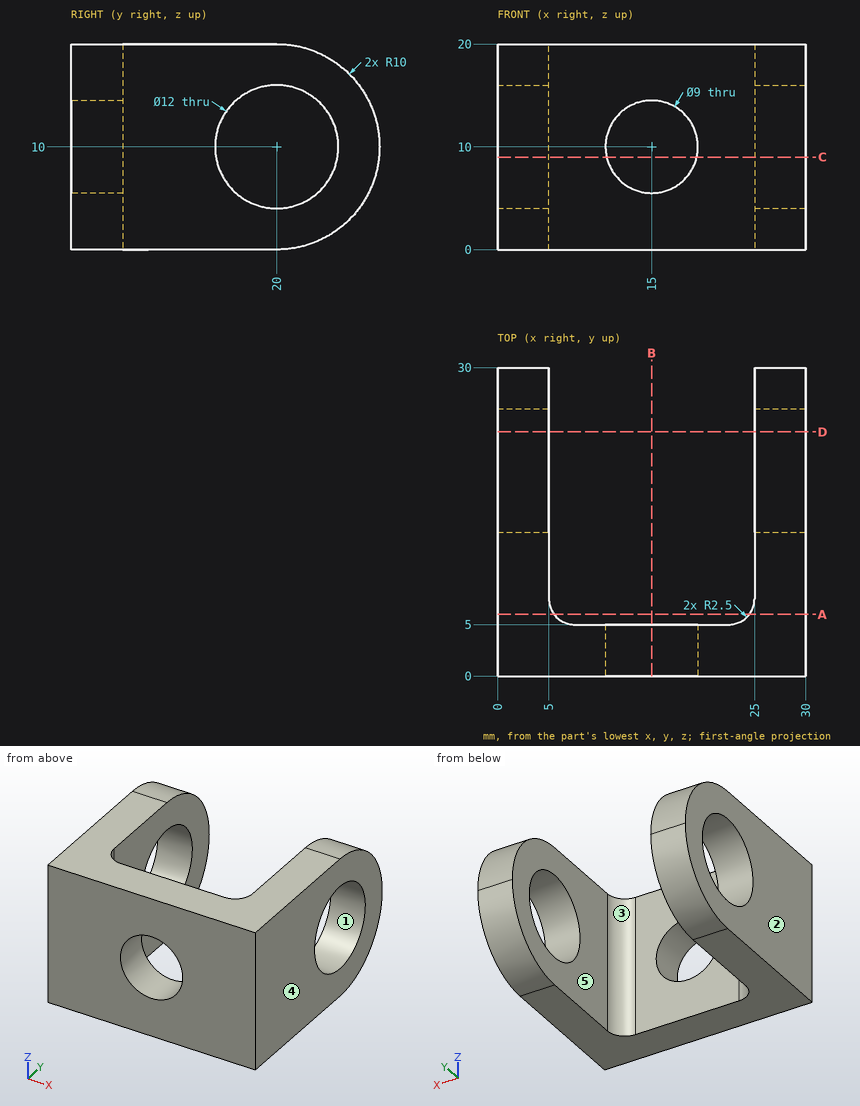
Job drawing, mm, ordinate dimensions from the low corner. One solid piece. A direction names the side the tool comes from. Give positions to 0.01 mm unless a question says otherwise; leave off trailing zeros. Write each loop counter-clockwise with the first axis right and the second up, starting at its lowest first coordinate (ties: lowest second). Pieces come first, ordered by that corner, then holes. Notation, with made-up numbers: (31, 30.25) -> (68, 30.25) arc R35 ccw to (68, 67.25) -> close; hole circle Ø7 at (-30.5, -14.75). An arc over 180 degrees is marked (long way). Return JSON: item names as keys, results as strings.
Item 1: Two-plate mould, pull along X, no slides. Class the marked faces 1, 2 and 3: +X half, -X half, draft (parallel to the pull), parting line (faces both ways), or undercut.
Answer below:
{"face 1": "draft", "face 2": "-X half", "face 3": "undercut"}
Item 2: Tool access for the marked faces 4 and 5: list every direction of +Z, -Z, +X, -X, +Y, -Y with a clear straight run to the whole face (end or side of a thin tool).
Answer below:
{"face 4": "+Z, -Z, +X, +Y, -Y", "face 5": "+Z, -Z, +Y"}
Item 3: Band-saw the part on A-A (y = 6). List the corners of the cut face in (x, z), then the cut area to 3 significant figures.
Answer below:
{"outline": "(0, 0) -> (5.5, 0) -> (5.5, 20) -> (0, 20) -> close; (24.5, 0) -> (30, 0) -> (30, 20) -> (24.5, 20) -> close", "area": "220 mm2"}
Item 4: Band-saw the part on C-C (z = 9). List the corners of the cut face in (x, y), then the cut area to 3 significant figures.
Answer below:
{"outline": "(0, 0) -> (10.61, 0) -> (10.61, 5) -> (7.5, 5) arc R2.5 cw to (5, 7.5) -> (5, 14.08) -> (0, 14.08) -> close; (0, 25.92) -> (5, 25.92) -> (5, 29.95) -> (0, 29.95) -> close; (19.39, 0) -> (30, 0) -> (30, 14.08) -> (25, 14.08) -> (25, 7.5) arc R2.5 cw to (22.5, 5) -> (19.39, 5) -> close; (25, 25.92) -> (30, 25.92) -> (30, 29.95) -> (25, 29.95) -> close", "area": "240 mm2"}
Item 5: Drill centre lines: probe 1 along Z at (x, y) = (15, 3.25); probe 2 along Y at (x, z) = (2.35, 10); probe 3 along Z at (x, y) = (1.9, 20). Where is each one in solid material? Low to high.
Answer below:
{"probe 1": "z = 0 to 5.5, 14.5 to 20", "probe 2": "y = 0 to 14, 26 to 30", "probe 3": "z = 0 to 4, 16 to 20"}
Item 6: Band-saw the part on B-B (x = 15). List the corners of the cut face in (y, z), then the cut area to 3 significant figures.
Answer below:
{"outline": "(0, 0) -> (5, 0) -> (5, 5.5) -> (0, 5.5) -> close; (0, 14.5) -> (5, 14.5) -> (5, 20) -> (0, 20) -> close", "area": "55.0 mm2"}
Item 7: Band-saw the part on D-D (y = 23.75). List the corners of the cut face in (x, z).
Answer below:
{"outline": "(0, 0.73) -> (5, 0.73) -> (5, 5.32) -> (0, 5.32) -> close; (0, 14.68) -> (5, 14.68) -> (5, 19.27) -> (0, 19.27) -> close; (25, 0.73) -> (30, 0.73) -> (30, 5.32) -> (25, 5.32) -> close; (25, 14.68) -> (30, 14.68) -> (30, 19.27) -> (25, 19.27) -> close"}
Item 8: Drop flat-ended pins along their axis: pin 1 (10.5 mm diameter, centred on x = 15, z = 10, fed in from +Y); pin 2 (10 mm diameter, centred on x = 9.5, z = 12, fed in from +Y); pin 3 (4 mm diameter, centred on x = 7.5, z = 11.5, fed in from +Y). Give the stop position or say it passes through.
Answer below:
{"pin 1": "stops at y = 5", "pin 2": "stops at y = 30", "pin 3": "stops at y = 6"}
